from build123d import *

# Parameters (mm, degrees)
SKICA1_W                     = 68
SKICA1_H                     = 48
SKICA1_R                     = 5.25
SKICA1_R_2                   = 3.05
P_IDAT_VYSUNUT_M1_DEPTH      = 2.5
SKICA2_W                     = 5
SKICA2_H                     = 5
P_IDAT_VYSUNUT_M2_DEPTH      = 7.6
SKICA3_R                     = 1.5
ODEBRAT_VYSUNUT_M1_DEPTH     = 10.1
SKICA8_R                     = 1.5
ODEBRAT_VYSUNUT_M2_DEPTH     = 10.1
SKICA9_R                     = 1.5
ODEBRAT_VYSUNUT_M3_DEPTH     = 10.1
SKICA10_R                    = 1.5
ODEBRAT_VYSUNUT_M4_DEPTH     = 10.1
P_IDAT_VYSUNUT_M3_DEPTH      = 8
P_IDAT_VYSUNUT_M3_DEPTH_BACK = 56
SKICA11_W                    = 10
SKICA11_H                    = 2.5
SKICA12_R                    = 2
ODEBRAT_VYSUNUT_M5_DEPTH     = 8
P_IDAT_START                 = 2.5
SKICA13_W                    = 10
SKICA13_H                    = 8
SKICA13_R                    = 2
P_IDAT_VYSUNUT_M4_DEPTH      = 2.5


with BuildPart() as part:
    # Skica1 → Přidat vysunutím1 (new body)
    with BuildSketch(Plane.XY):
        Rectangle(SKICA1_W, SKICA1_H)
        with Locations((-14, 0)):
            Circle(SKICA1_R, mode=Mode.SUBTRACT)
        with Locations((14, 0)):
            Circle(SKICA1_R_2, mode=Mode.SUBTRACT)
    extrude(amount=P_IDAT_VYSUNUT_M1_DEPTH)

    # Skica2 → Přidat vysunutím2 (add)
    with BuildSketch(Plane.XY.offset(2.5)):
        with Locations((-31.5, 21.5)):
            Rectangle(SKICA2_W, SKICA2_H)
        with Locations((31.5, 21.5)):
            Rectangle(SKICA2_W, SKICA2_H)
        with Locations((31.5, -21.5)):
            Rectangle(SKICA2_W, SKICA2_H)
        with Locations((-31.5, -21.5)):
            Rectangle(SKICA2_W, SKICA2_H)
    extrude(amount=P_IDAT_VYSUNUT_M2_DEPTH)

    # Skica3 → Odebrat vysunutím1 (cut)
    with BuildSketch(Plane.XY.offset(10.1)):
        with Locations((-31.5, 21.5)):
            Circle(SKICA3_R)
    extrude(amount=-ODEBRAT_VYSUNUT_M1_DEPTH, mode=Mode.SUBTRACT)

    # Skica8 → Odebrat vysunutím2 (cut)
    with BuildSketch(Plane.XY.offset(10.1)):
        with Locations((31.5, 21.5)):
            Circle(SKICA8_R)
    extrude(amount=-ODEBRAT_VYSUNUT_M2_DEPTH, mode=Mode.SUBTRACT)

    # Skica9 → Odebrat vysunutím3 (cut)
    with BuildSketch(Plane.XY.offset(10.1)):
        with Locations((31.5, -21.5)):
            Circle(SKICA9_R)
    extrude(amount=-ODEBRAT_VYSUNUT_M3_DEPTH, mode=Mode.SUBTRACT)

    # Skica10 → Odebrat vysunutím4 (cut)
    with BuildSketch(Plane.XY.offset(10.1)):
        with Locations((-31.5, -21.5)):
            Circle(SKICA10_R)
    extrude(amount=-ODEBRAT_VYSUNUT_M4_DEPTH, mode=Mode.SUBTRACT)

    # Skica11 → Přidat vysunutím3 (add, two sides: drawn at the far end of the back side and taken through both)
    with BuildSketch(Plane(origin=(0, 24, 0), x_dir=(1, 0, 0), z_dir=(0, 1, 0)).offset(-P_IDAT_VYSUNUT_M3_DEPTH_BACK)):
        with Locations((-29, -1.25)):
            Rectangle(SKICA11_W, SKICA11_H)
        with Locations((29, -1.25)):
            Rectangle(SKICA11_W, SKICA11_H)
    extrude(amount=P_IDAT_VYSUNUT_M3_DEPTH + P_IDAT_VYSUNUT_M3_DEPTH_BACK)

    # Skica12 → Odebrat vysunutím5 (cut)
    with BuildSketch(Plane.XY.offset(2.5)):
        with Locations((-29, 28)):
            Circle(SKICA12_R)
        with Locations((29, 28)):
            Circle(SKICA12_R)
        with Locations((29, -28)):
            Circle(SKICA12_R)
        with Locations((-29, -28)):
            Circle(SKICA12_R)
    extrude(amount=-ODEBRAT_VYSUNUT_M5_DEPTH, mode=Mode.SUBTRACT)

    # Skica13 → Přidat vysunutím4 (add)
    # profile 1 of 4: a face of its own
    with BuildSketch(Plane.XY.offset(2.5).offset(P_IDAT_START)):
        with Locations((-29, 28)):
            Rectangle(SKICA13_W, SKICA13_H)
        with Locations((-29, 28)):
            Circle(SKICA13_R, mode=Mode.SUBTRACT)
    # profile 2 of 4: a face of its own
    with BuildSketch(Plane.XY.offset(2.5).offset(P_IDAT_START)):
        with Locations((29, 28)):
            Rectangle(SKICA13_W, SKICA13_H)
        with Locations((29, 28)):
            Circle(SKICA13_R, mode=Mode.SUBTRACT)
    # profile 3 of 4: a face of its own
    with BuildSketch(Plane.XY.offset(2.5).offset(P_IDAT_START)):
        with Locations((29, -28)):
            Rectangle(SKICA13_W, SKICA13_H)
        with Locations((29, -28)):
            Circle(SKICA13_R, mode=Mode.SUBTRACT)
    # profile 4 of 4: a face of its own
    with BuildSketch(Plane.XY.offset(2.5).offset(P_IDAT_START)):
        with Locations((-29, -28)):
            Rectangle(SKICA13_W, SKICA13_H)
        with Locations((-29, -28)):
            Circle(SKICA13_R, mode=Mode.SUBTRACT)
    extrude(amount=-P_IDAT_VYSUNUT_M4_DEPTH)


solid = part.part
Could you check a few things on this model? Use its own coordinates, in mm. A direction names the side the tool comes from. Give positions to 0.01 mm unless a question says otherwise; leave off trailing zeros. Loops run counter-clockwise (first coordinate to the right, second up) from the corner with the lowest first, then second, coordinate; pieces in that order, holes last. Notation, with made-up numbers: (-10, -37) -> (18, -37) arc R37 ccw to (18, 2) -> close; hole circle Ø3 at (69.25, -39). An arc over 180 degrees is marked (long way). Answer as CSV lines item,"result". Start each with the question number.
(1) Which directions (+Z, -Z, +X, -X, +Y, -Y) give clear straight access to the entire face, cutting with the end or side of a thin tool? Please do faces 4 (the flat face through (-32, 19, 6)), 5 (the flat face through (24, -28, 3)), 6 (the flat face through (26, 24, 4)).
(2) If we section it at B-B on y = 0: Write out the boundary of the cut face in (x, z), then the cut area to 4 significant figures.
(3) I need wall thicknesses on probe 1 along Y at (x, z) = (31.5, 5.5); probe 2 along Y at (x, z) = (-26.5, 3); probe 3 along Y at (x, z) = (14, 0.85). Which ranges of each line are inside material? Lowest first, please.
(4) If we section it at A-A on z = 6.5: Write out the boundary of the cut face in (x, y), then the cut area to 3 significant figures.
(5) If we section it at C-C on z = 1: Write out the boundary of the cut face in (x, y), then the cut area to 3 significant figures.
(6) We'd pull the mould along X, two halves only. Please class faces 1 (the flat face through (24, 28, 3)), 2 (the flat face through (0, -24, 1)), 3 (the flat face through (0, 0, 0)): released by +X, released by -X, zero draft, split by the parting line, or undercut.
(7) I'm going to push flat-ended pins straight in: pin 1 Ø3.5 at (x, y) = (31, 21.5) entering from +Z; pin 2 Ø2.5 at (x, y) = (31.5, -21.5) entering from +Z; pin 3 Ø1.5 at (x, z) = (30.5, 7) entering from -Y; pin 4 Ø5.5 at (x, y) = (14, 0) entering from -Z. Where does each tip first touch, or does it pass through?
(8) If we section it at D-D on x = -14: Write out the boundary of the cut face in (y, z), then the cut area to 4 significant figures.
Computed:
1,face 4,"+Z, +X, -X"
1,face 5,"+Z, -Z, -Y"
1,face 6,"+Z"
2,outline,"(-34, 0) -> (-19.25, 0) -> (-19.25, 2.5) -> (-34, 2.5) -> close; (-8.75, 0) -> (10.95, 0) -> (10.95, 2.5) -> (-8.75, 2.5) -> close; (17.05, 0) -> (34, 0) -> (34, 2.5) -> (17.05, 2.5) -> close"
2,area,"128.5 mm2"
3,probe 1,"y = -24 to -23, -20 to -19, 19 to 20, 23 to 24"
3,probe 2,"y = -32 to -24, 24 to 32"
3,probe 3,"y = -24 to -3.05, 3.05 to 24"
4,outline,"(-34, -24) -> (-29, -24) -> (-29, -19) -> (-34, -19) -> close; (-34, 19) -> (-29, 19) -> (-29, 24) -> (-34, 24) -> close; (29, -24) -> (34, -24) -> (34, -19) -> (29, -19) -> close; (29, 19) -> (34, 19) -> (34, 24) -> (29, 24) -> close; hole circle Ø3 at (-31.5, -21.5); hole circle Ø3 at (-31.5, 21.5); hole circle Ø3 at (31.5, -21.5); hole circle Ø3 at (31.5, 21.5)"
4,area,"71.7 mm2"
5,outline,"(-34, -32) -> (-24, -32) -> (-24, -24) -> (24, -24) -> (24, -32) -> (34, -32) -> (34, 32) -> (24, 32) -> (24, 24) -> (-24, 24) -> (-24, 32) -> (-34, 32) -> close; hole circle Ø4 at (-29, -28); hole circle Ø4 at (-29, 28); hole circle Ø10.5 at (-14, 0); hole circle Ø6.1 at (14, 0); hole circle Ø4 at (29, -28); hole circle Ø4 at (29, 28)"
5,area,"3,420 mm2"
6,face 1,"undercut"
6,face 2,"undercut"
6,face 3,"zero draft"
7,pin 1,"stops at z = 10.1"
7,pin 2,"stops at z = 2.5"
7,pin 3,"stops at y = -24"
7,pin 4,"passes through"
8,outline,"(-24, 0) -> (-5.25, 0) -> (-5.25, 2.5) -> (-24, 2.5) -> close; (5.25, 0) -> (24, 0) -> (24, 2.5) -> (5.25, 2.5) -> close"
8,area,"93.75 mm2"
